Work out the finished part from the listing and answer in its coordinate system (mm). A direction names the side the tool comes from. Round coordinates to 2 decimals unless told otherwise and drop trailing zeros. Order: outer loops, then holes, each group sorted by start corner. A loop starts at its lowest first (then second) coordinate and runs counter-clockwise, first axis right, second up. Notation, with made-up numbers: (1.25, 41) -> (58.25, 41) arc R21 cw to (58.25, 53) -> close; hole circle Ø11 at (20, 29.5). An arc over 180 degrees is marked (long way). Use a Markdown table: item, result. Add a question column.
Item 1: For a pull along Y with two mould halves and no side action, classify faces 1 (the flat face through (13, 0, 28)), 2 (the cylindrical face through (0, 127, 8)), 3 (the cylindrical face through (11.99, 0.53, 13.8)) as +Y half, -Y half, draft (parallel to the pull), parting line (faces both ways), or undercut.
Item 2: A cutting plane is placed at B-B, the plane x = 0. Determine the outline of the cut face in (y, z), plus the area to 3 significant figures.
Item 3: A cutting plane is placed at A-A, the plane y = 0. Determine the outline of the cut face in (x, z).
Item 4: Find the intervals of material crossed by L1, parallel to Y at x = 0, z = 11.75; L2, parallel to Y at x = 0, z = 20; L3, parallel to Y at x = -8, z = 18.25, in increasing order. Write a range as [from, to].
Item 5: A cutting plane is placed at C-C, the plane x = 23. Determine the outline of the cut face in (y, z), plus the area to 3 significant figures.
Item 6: A tool of negligible diameter and unlimited length cuts with its end or side. For faces 4 (the flat face through (24.967, 57.933, 7.888)), 5 (the flat face through (3, 107, 23)), 6 (the flat face through (0, 47, 16)), from which of +Z, -Z, +X, -X, +Y, -Y can it reach the whole face along a straight path? Write none if from no direction.
Item 7: Flat-ended cylindrical pins translate along their axes: P1, Ø20, axis at x = -5, y = 106, coming from the +Z side; P2, Ø1, axis at x = -9.5, z = 5.5, coming from the +Y side; P3, Ø12, axis at y = 86, z = 14.5, coming from the -X side. Find the tip coordinate at first contact, or state that the pin passes through.
Item 8: A cutting plane is placed at D-D, the plane y = -21. Determine the outline of the cut face in (x, z).
from build123d import *

# Parameters (mm, degrees)
F1_DEPTH = 16
F2_R     = 12.5
F2_R_2   = 30
F3_DEPTH = 12
F5_D     = 24
F7_D     = 11
F8_R     = 12.5
F9_DEPTH = 5


with BuildPart() as f1:
    # F0 (on Top) → F1 (new body)
    with BuildSketch(Plane.XY):
        with BuildLine():
            Line((-14.763017, 114.655808), (-33.669786, 9.557486))
            Line((-33.669786, 9.557486), (-34.88973, 2.776097))
            ThreePointArc((-34.88973, 2.776097), (0, -35), (34.88973, 2.776097))
            Line((34.88973, 2.776097), (14.763017, 114.655808))
            ThreePointArc((14.763017, 114.655808), (0, 127), (-14.763017, 114.655808))
        make_face()
    extrude(amount=F1_DEPTH)

    # F2 (on face) → F3 (join)
    with BuildSketch(Plane.XY.offset(16)):
        with Locations((0, 112)):
            Circle(F2_R)
        Circle(F2_R_2)
    extrude(amount=F3_DEPTH)

    # F5 (through all)
    with Locations(Plane.XY.offset(28)):
        with Locations((0, 0)):
            Hole(F5_D / 2)

    # F7 (through all)
    with Locations(Plane.XY.offset(28)):
        with Locations((0, 112)):
            Hole(F7_D / 2)

    # F8 (on face) → F9 (cut)
    with BuildSketch(Plane.XY.offset(28)):
        with Locations((0, 112)):
            Circle(F8_R)
    extrude(amount=-F9_DEPTH, mode=Mode.SUBTRACT)


solid = f1.part
Reported:
| question | item | result |
|---|---|---|
| 1 | face 1 | draft |
| 1 | face 2 | +Y half |
| 1 | face 3 | undercut |
| 2 | outline | (-35, 0) -> (-12, 0) -> (-12, 28) -> (-30, 28) -> (-30, 16) -> (-35, 16) -> close; (12, 0) -> (106.5, 0) -> (106.5, 23) -> (99.5, 23) -> (99.5, 16) -> (30, 16) -> (30, 28) -> (12, 28) -> close; (117.5, 0) -> (127, 0) -> (127, 16) -> (124.5, 16) -> (124.5, 23) -> (117.5, 23) -> close |
| 2 | area | 2,560 mm² |
| 3 | outline | (-35, 0) -> (-12, 0) -> (-12, 28) -> (-30, 28) -> (-30, 16) -> (-35, 16) -> close; (12, 0) -> (35, 0) -> (35, 16) -> (30, 16) -> (30, 28) -> (12, 28) -> close |
| 4 | L1 | [-35, -12], [12, 106.5], [117.5, 127] |
| 4 | L2 | [-30, -12], [12, 30], [99.5, 106.5], [117.5, 124.5] |
| 4 | L3 | [-28.91, -8.94], [8.94, 28.91], [102.4, 121.6] |
| 5 | outline | (-26.38, 0) -> (68.87, 0) -> (68.87, 16) -> (19.26, 16) -> (19.26, 28) -> (-19.26, 28) -> (-19.26, 16) -> (-26.38, 16) -> close |
| 5 | area | 1,990 mm² |
| 6 | face 4 | +Z, -Z, +X, +Y |
| 6 | face 5 | +Z, +X, -X, +Y |
| 6 | face 6 | +Z |
| 7 | P1 | z = 23 |
| 7 | P2 | y = 124 |
| 7 | P3 | x = -21 |
| 8 | outline | (-28, 0) -> (28, 0) -> (28, 16) -> (21.42, 16) -> (21.42, 28) -> (-21.42, 28) -> (-21.42, 16) -> (-28, 16) -> close |
